Work out the finished part from the listing and answer in its coordinate system (mm). A direction names the side the tool comes from. Coordinates: 2 decimals unless noted, no trailing zeros. Write each loop counter-clockwise with the first axis right and the second up, starting at its lowest first coordinate (ties: lowest second). Pieces come first, ordered by that corner, then holes. Notation, with made-up numbers: M 40.5,42 L 65.5,42 A22 ccw 65.5,56 Z; hole C 22.5,68.25 d11. An arc over 180 degrees is marked long. Answer as CSV lines item,"result". Start each with the question number.
(1) A cutting plane is placed at B-B on x = -2.25. Give the vertices of the cut face in (y, z), then the cut area to 3 significant figures.
(2) For faces 1 (the flat face through (-5.234, -2, 19)), 2 (the flat face through (-7, 0, 20)), 3 (the flat face through (-14, -2, 16.768)), determine the directions among +Z, -Z, +X, -X, +Y, -Y from which every point of the face is accessible in a straight line to the end or side of a thin tool.
(3) Find the intervals of material crossed by L1, parallel to X at y = -3.25, z = 23.5; L2, parallel to X at y = -3.5, z = 29.25; L3, parallel to Z at x = -5, y = -2.4, in increasing order. Write a range as [from, to].
(4) Flat-ended cylindrical pins translate along their axes: P1, Ø2.5, axis at x = -5.5, y = -2.5, coming from the +Z side; P2, Ø1.5, axis at y = -2, z = 20, coming from the -X side; P3, Ø1.5, axis at y = -2, z = 29, coming from the -X side. Find the tip coordinate at first contact, or state that the pin passes through.
(5) A cutting plane is placed at A-A on z = 13.5. Give the vertices of the cut face in (x, y), then the cut area to 3 significant figures.
(6) The mould has two halves that part along X. Classify faces 4 (the flat face through (1, -2, 30.708)), 5 (the flat face through (-8.484, -2, 20)), 6 (the cylindrical face through (-10, -2, 10)): released by +X, released by -X, zero draft, split by the parting line, or undercut.
(7) A cutting plane is placed at C-C on z = 18.5. Give the vertices of the cut face in (x, y), then the cut area to 4 significant figures.
from build123d import *

# Parameters (mm, degrees)
F1_DEPTH    = 5
F2_R        = 2
F3_DEPTH    = 2
F4_T1_DEPTH = 11
F4_T3_DEPTH = 6.0917941426


# Not quite as in the source:
# - a fillet or chamfer that OpenCascade refuses, or shapes differently, is made with other operations: its cross-section is extruded or revolved along the edge and cut away or added


with BuildPart() as f1:
    # F0 (on Front) → F1 (new body)
    with BuildSketch(Plane.XZ):
        with BuildLine():
            Line((1.4157007724, 23.5682009265), (1.4157007724, 30.7082009265))
            Line((1.4157007724, 30.7082009265), (0, 30.7082009265))
            Line((0, 30.7082009265), (0, 29.0815811604))
            Line((0, 29.0815811604), (0, 25.7029440254))
            Line((0, 25.7029440254), (-8.4842955694, 25.7029440254))
            Line((-8.4842955694, 25.7029440254), (-8.4842955694, 14.7682009265))
            ThreePointArc((-8.4842955694, 14.7682009265), (-9.7762482479, 12.7647114857), (-11.0682009265, 14.7682009265))
            Line((-11.0682009265, 14.7682009265), (-14.7682009265, 14.7682009265))
            ThreePointArc((-14.7682009265, 14.7682009265), (-10.001250077, 10.001250077), (-5.2342992276, 14.7682009265))
            Line((-5.2342992276, 14.7682009265), (-5.2342992276, 23.5682009265))
            Line((-5.2342992276, 23.5682009265), (1.4157007724, 23.5682009265))
        make_face()
    extrude(amount=F1_DEPTH)

    # F2
    f2_edges = [f1.edges().sort_by_distance(p)[0] for p in [
        (1.415701, -2.5, 23.568201),
    ]]
    fillet(f2_edges, radius=F2_R)

    # F3 (add): a face of the model
    f3_faces = [f1.faces().sort_by_distance(p)[0] for p in [
        (-12.9182009265, -2.5, 14.7682009265),
    ]]
    extrude(f3_faces, amount=F3_DEPTH)

    # F4: fillet of radius 1.2 on 2 edges, made by hand

    # F4_s2 → F4_t1 (cut)
    with BuildSketch(Plane.XZ.offset(-3)):
        with BuildLine():
            add(Edge.make_bspline(
                [(-11.0682009265, 15.5682009265), (-11.0682009265, 16.7682009265), (-12.2682009265, 16.7682009265)],
                knots=[0, 0, 0, 1, 1, 1], degree=2, weights=[1, 1, 1]))
            Line((-12.2682009265, 16.7682009265), (-11.0682009265, 16.7682009265))
            Line((-11.0682009265, 16.7682009265), (-11.0682009265, 15.5682009265))
        make_face()
    extrude(amount=F4_T1_DEPTH, mode=Mode.SUBTRACT)

    # F4_s4 → F4_t3 (cut)
    with BuildSketch(Plane.XZ.offset(-0.5458970713)):
        with BuildLine():
            add(Edge.make_bspline(
                [(-11.1261089729, 14.6182854421), (-11.0682009265, 14.7978698213), (-11.0682009265, 14.986559755)],
                knots=[0, 0, 0, 1, 1, 1], degree=2, weights=[1, 1, 1]))
            Line((-11.0682009265, 14.986559755), (-11.0682009265, 14.7682009265))
            ThreePointArc((-11.0682009265, 14.7682009265), (-11.0992800608, 14.6940640537), (-11.1261089729, 14.6182854421))
        make_face()
    extrude(amount=F4_T3_DEPTH, mode=Mode.SUBTRACT)


solid = f1.part
Here are the results:
1,outline,"M -5,23.57 L 0,23.57 L 0,25.7 L -5,25.7 Z"
1,area,"10.7 mm^2"
2,face 1,"-Z, +X, +Y, -Y"
2,face 2,"+Z, -Z, +X, -X, +Y"
2,face 3,"+Z, -X, +Y, -Y"
3,L1,"x = [-8.48, -5.23]"
3,L2,"x = [0, 1.42]"
3,L3,"z = [23.57, 25.7]"
4,P1,"stops at z = 25.7"
4,P2,"stops at x = -8.48"
4,P3,"stops at x = 0"
5,outline,"M -14.6,-5 L -11.02,-5 L -11.02,0 L -14.6,0 Z; M -8.53,-5 L -5.41,-5 L -5.41,0 L -8.53,0 Z"
5,area,"33.5 mm^2"
6,face 4,"zero draft"
6,face 5,"undercut"
6,face 6,"split by the parting line"
7,outline,"M -8.48,-5 L -5.23,-5 L -5.23,0 L -8.48,0 Z"
7,area,"16.25 mm^2"
